from build123d import *

# Parameters (mm, degrees)
SKETCH_2_W               = 30
SKETCH_2_H               = 30
EXTRUDE_1_DEPTH          = 100
SKETCH_3_W               = 18
SKETCH_3_H               = 18
EXTRUDE_2_DEPTH          = 35
PATTERN_CIRCULAR_1_COUNT = 2
SKETCH_4_R               = 10.254249717
EXTRUDE_4_DEPTH          = 5
SKETCH_5_R               = 5
CUT_EXTRUDE_2_DEPTH      = 15
PATTERN_CIRCULAR_3_COUNT = 2
PATTERN_CIRCULAR_4_COUNT = 2


with BuildPart() as part:
    # 草图2 → 凸台-拉伸1 (new body)
    with BuildSketch(Plane.XY):
        Rectangle(SKETCH_2_W, SKETCH_2_H)
    extrude(amount=EXTRUDE_1_DEPTH)

    # 草图3 → 凸台-拉伸2 (add)
    with BuildSketch(Plane(origin=(15, 0, 0), x_dir=(0, 0, -1), z_dir=(1, 0, 0))):
        with Locations((-84.019000904, 0)):
            Rectangle(SKETCH_3_W, SKETCH_3_H)
    extrude_2 = extrude(amount=EXTRUDE_2_DEPTH)

    # 阵列(圆周)1: 凸台-拉伸2 ×2 about axis
    pattern_circular_1_axis = Axis((0, 0, 0), (0, 0, 1))
    for i in range(1, PATTERN_CIRCULAR_1_COUNT):
        add(extrude_2.rotate(pattern_circular_1_axis, i * 360 / PATTERN_CIRCULAR_1_COUNT))

    # 草图4 → 凸台-拉伸4 (add)
    with BuildSketch(Plane(origin=(0, 15, 0), x_dir=(1, 0, 0), z_dir=(0, 1, 0))):
        with Locations((0, -26.28538531)):
            Circle(SKETCH_4_R)
    extrude_4 = extrude(amount=EXTRUDE_4_DEPTH)

    # 草图5 → 切除-拉伸2 (cut)
    with BuildSketch(Plane(origin=(0, 20, 0), x_dir=(1, 0, 0), z_dir=(0, 1, 0))):
        with Locations((0, -26.28538531)):
            Circle(SKETCH_5_R)
    cut_extrude_2 = extrude(amount=-CUT_EXTRUDE_2_DEPTH, mode=Mode.SUBTRACT)

    # 阵列(圆周)3: 凸台-拉伸4 ×2 about axis
    pattern_circular_3_axis = Axis((0, 0, 100), (0, 0, -1))
    for i in range(1, PATTERN_CIRCULAR_3_COUNT):
        add(extrude_4.rotate(pattern_circular_3_axis, i * 360 / PATTERN_CIRCULAR_3_COUNT))

    # 阵列(圆周)4: 切除-拉伸2 ×2 about axis
    pattern_circular_4_axis = Axis((0, 0, 100), (0, 0, -1))
    for i in range(1, PATTERN_CIRCULAR_4_COUNT):
        add(cut_extrude_2.rotate(pattern_circular_4_axis, i * 360 / PATTERN_CIRCULAR_4_COUNT), mode=Mode.SUBTRACT)


solid = part.part
Build history of the part. All positions in model axes, mm. A direction names the side the tool comes from. Give positions to 0.01 mm unless a question says otherwise; leave off trailing zeros. Order: outer loops, then holes, each group sorted by start corner. A loop starts at its lowest first (then second) coordinate and runs counter-clockwise, first axis right, second up. Notation, with made-up numbers: M -25.5,71 L -5.5,71 A26 cw -5.5,101 Z; hole C -14.75,-13 d5. An arc over 180 degrees is marked long. Put each result on its own line as item: value.
Item 1: Probe line 1 (Z direction, x = 0, y = -16); line 2 (Y direction, x = 5, z = 14.5); line 3 (Z direction, x = 41.5, y = -4). List the from-to ranges inside material, lowest first. Write a range as [from, to].
From the geometry:
line 1: z = [16.03, 21.29], [31.29, 36.54]
line 2: y = [-15, 15]
line 3: z = [75.02, 93.02]
Item 2: 3-axis set-ups, long thin cutter, end or side, ignore diameter. For faces 1 (the flat face through (-32, -9, 84)), 2 (the flat face through (-32, 0, 75.019)), 3 (the flat face through (-32, 9, 84)): which of +Z, -Z, +X, -X, +Y, -Y reach the whole face in a straight line?
From the geometry:
face 1: +Z, -Z, -X, -Y
face 2: -Z, -X, +Y, -Y
face 3: +Z, -Z, -X, +Y
Item 3: Slice it at B-B, the plane x = 0. Write the cut outline in (y, z), plus the area to 3 significant figures.
From the geometry:
outline: M -20,16.03 L -15,16.03 L -15,0 L 15,0 L 15,16.03 L 20,16.03 L 20,21.29 L 5,21.29 L 5,31.29 L 20,31.29 L 20,36.54 L 15,36.54 L 15,100 L -15,100 L -15,36.54 L -20,36.54 L -20,31.29 L -5,31.29 L -5,21.29 L -20,21.29 Z
area: 2,910 mm2
Item 4: Flat gauge pins, fed straight in: pin 1 Ø5.5 at (x, y) = (38.5, -2.5) entering from +Z; pin 2 Ø6 at (y, z) = (11, 18.5) entering from +X; pin 3 Ø11 at (x, z) = (-2, 25.5) entering from +Y; pin 4 Ø9 at (x, y) = (-31.5, 1) entering from -Z. Where does each tip first touch, or does it go through?
From the geometry:
pin 1: stops at z = 93.02
pin 2: stops at x = 15
pin 3: stops at y = 20
pin 4: stops at z = 75.02
Item 5: Slice it at A-A, the plane z = 90. Write the cut outline in (x, y), plus the area to 3 significant figures.
From the geometry:
outline: M -50,-9 L -15,-9 L -15,-15 L 15,-15 L 15,-9 L 50,-9 L 50,9 L 15,9 L 15,15 L -15,15 L -15,9 L -50,9 Z
area: 2,160 mm2
Item 6: Slice it at C-C, the plane y = 2. Write the cut outline in (x, z), plus the area to 3 significant figures.
From the geometry:
outline: M -50,75.02 L -15,75.02 L -15,0 L 15,0 L 15,75.02 L 50,75.02 L 50,93.02 L 15,93.02 L 15,100 L -15,100 L -15,93.02 L -50,93.02 Z
area: 4,260 mm2
Item 7: Two-plate mould, pull along X, no slides. Class faces 4 (the flat face through (-2.14, -20, 21.58)), 5 (the cylindrical face through (-5.513, -17.465, 17.639)), 6 (the cylindrical face through (-1.084, 12.605, 31.166)): +X half, -X half, draft (parallel to the pull), parting line (faces both ways), or undercut.
From the geometry:
face 4: draft
face 5: parting line
face 6: undercut
Item 8: Slice it at D-D, the plane y = -18. Write the cut outline in (x, z).
From the geometry:
outline: C 0,26.29 d20.51; hole C 0,26.29 d10
